For this review, use the dimensioned drawing (mm, ordinates from the lowest corner) and the shaded views. A direction names the side the tool comes from. Round coordinates to 2 decimals unless told otherwise and drop trailing zeros. Write each loop counter-clockwise with the first axis right and the second up, starting at its lowest first coordinate (ties: lowest second). Pieces come first, ordered by that corner, then holes. Notation, with made-up numbers: M 10.5,88.5 L 42.5,88.5 A23 ccw 42.5,120.5 Z; hole C 62.25,59.25 d3. An arc over 180 degrees is marked long. One line per question, with ' | ' between items.
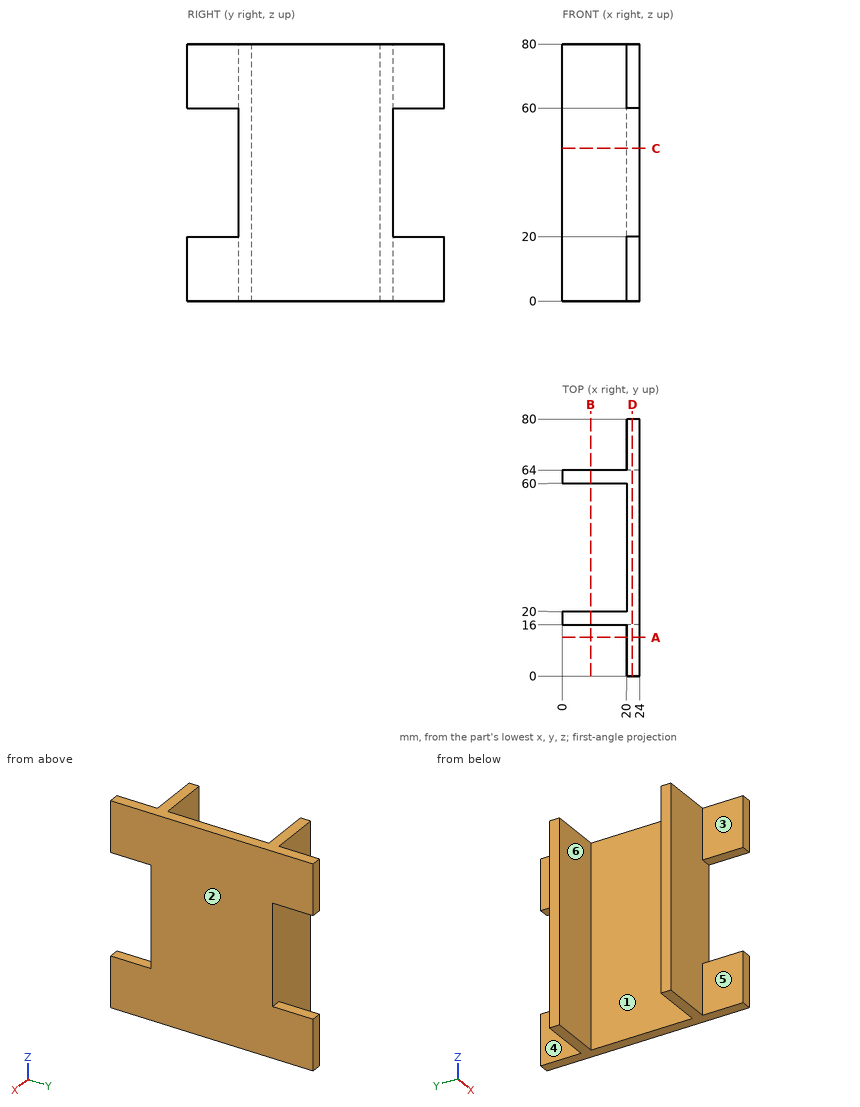
Item 1: Insertion check: pin 1 Ø5 at (y, z) = (7.5, 11.5) entering from -X; pin 2 Ø3 at (x, z) = (8.5, 37) entering from +Y; pin 3 Ø6 at (x, z) = (13.5, 29.5) entering from -Y. Each pin has a flat end and moves straight along its axis. Give the tip position at first contact, or say it passes through.
Results:
pin 1: x = 20 | pin 2: y = 64 | pin 3: y = 16
Item 2: Machinability: for the marked faces 1, 2, 3 and 4, which of the approach directions +Z, -Z, +X, -X, +Y, -Y give a long, thin tool a straight path to every point of the face, cutting with its end or side? Answer none if there is none.
Results:
face 1: +Z, -Z, -X | face 2: +Z, -Z, +X, +Y, -Y | face 3: +Z, -Z, -X, -Y | face 4: +Z, -Z, -X, +Y
Item 3: Take a section at A-A (y = 12). Write out the cut boundary in (x, z).
Results:
outline: M 20,0 L 24,0 L 24,20 L 20,20 Z; M 20,60 L 24,60 L 24,80 L 20,80 Z
Item 4: Take a section at B-B (x = 8.75). Write out the cut boundary in (y, z).
Results:
outline: M 16,0 L 20,0 L 20,80 L 16,80 Z; M 60,0 L 64,0 L 64,80 L 60,80 Z
Item 5: To check wall thickness, follow line 1 along Y through (x, z) = (17.5, 73); line 2 along Z through (x, y) = (23.25, 72); line 3 along X through (y, z) = (72.5, 75). State the ranges of each line that lie inside material, in increasing order. Write a range as from..to.
Results:
line 1: 16..20, 60..64 | line 2: 0..20, 60..80 | line 3: 20..24
Item 6: Take a section at D-D (x = 21.75). Write out the cut boundary in (y, z), then the cut area to 3 significant figures.
Results:
outline: M 0,0 L 80,0 L 80,20 L 64,20 L 64,60 L 80,60 L 80,80 L 0,80 L 0,60 L 16,60 L 16,20 L 0,20 Z | area: 5,120 mm2
Item 7: Take a section at C-C (z = 47.5). Write out the cut boundary in (x, y), then the cut area to 3 significant figures.
Results:
outline: M 0,16 L 24,16 L 24,64 L 0,64 L 0,60 L 20,60 L 20,20 L 0,20 Z | area: 352 mm2
Item 8: Mouldability with a two-part tool opening along Y and no side actions: class the marked faces 5 and 6 as +Y half, -Y half, draft (parallel to the pull), parting line (faces both ways), or undercut.
Results:
face 5: draft | face 6: undercut
